```python
from build123d import *

# Parameters (mm, degrees)
SKETCH1_R           = 7.5
SKETCH1_R_2         = 4
BOSS_EXTRUDE1_DEPTH = 30
SKETCH4_R           = 2
CUT_EXTRUDE1_DEPTH  = 19


with BuildPart() as part:
    # Sketch1 → Boss-Extrude1 (new body)
    with BuildSketch(Plane.XY):
        Polygon((6.7, 11.09607963), (17, 11.09607963), (17, 5.09607963), (16.2, 3.09607963), (16.2, -5.843260198), (15.139339828, -6.90392037), (7.024607597, -6.90392037), (3.5, -10.90392037), (0, -10.90392037), (-3.5, -10.90392037), (-7.024607597, -6.90392037), (-15.139339828, -6.90392037), (-16.2, -5.843260198), (-16.2, 3.09607963), (-17, 5.09607963), (-17, 11.09607963), (-6.7, 11.09607963), (-6, 10.39607963), (6, 10.39607963), align=None)
        Circle(SKETCH1_R, mode=Mode.SUBTRACT)
        Circle(SKETCH1_R)
        Circle(SKETCH1_R_2, mode=Mode.SUBTRACT)
    extrude(amount=BOSS_EXTRUDE1_DEPTH)

    # Sketch4 → Cut-Extrude1 (cut, through all)
    with BuildSketch(Plane.XZ.offset(6.90392037)):
        with Locations((-12, 24)):
            Circle(SKETCH4_R)
        with Locations((-12, 6)):
            Circle(SKETCH4_R)
        with Locations((12, 6)):
            Circle(SKETCH4_R)
        with Locations((12, 24)):
            Circle(SKETCH4_R)
    extrude(amount=-CUT_EXTRUDE1_DEPTH, mode=Mode.SUBTRACT)


solid = part.part
```
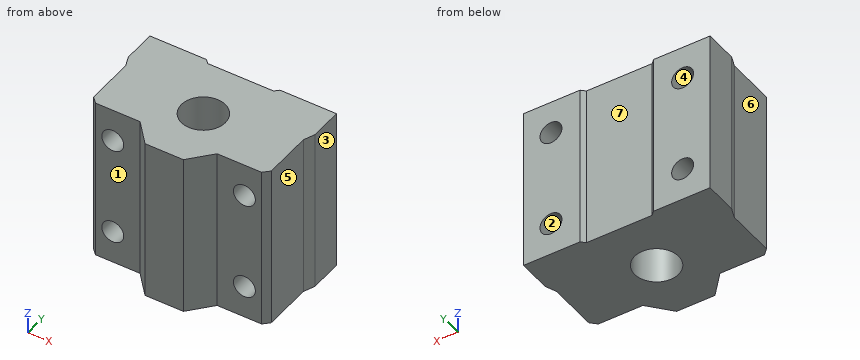
CAD build for the part. Positions are in the model's coordinates, mm. Face numbers are marked on the shaded views. A direction names the side the tool comes from. Round coordinates to 2 decimals unless told otherwise and drop trailing zeros. Loops run counter-clockwise (first coordinate to the right, second up) from the corner with the lowest first, then second, coordinate; pieces in that order, holes last. Notation, with made-up numbers: M 60,33.25 L 105,33.25 A17 ccw 105,59.25 Z; hole C 46,32 d2. An arc over 180 degrees is marked long. Return JSON: item names as keys, results as strings. Group by question number.
(1) Drop flat-ended pins along their axis: P1, Ø12, axis at y = -2.5, z = 6, coming from the +X side; P2, Ø2.5, axis at x = -10, z = 22, coming from the -Y side; P3, Ø1, axis at x = -1.5, z = 27, coming from the +Y side. Give the stop position or say it passes through.
(2) Saw through at D-D, the plane y = 7.75. List the corners of the cut face in (x, z), and give its area (3 significant figures).
(3) Mould opens along X. For the marked faces 1, 2, 3 and 4 say: +X half, -X half, draft (parallel to the pull), parting line (faces both ways), or undercut.
(4) Saw through at B-B, the plane y = 0. List the corners of the cut face in (x, z), and give its area (3 significant figures).
(5) Saw through at A-A, the plane z = 6. List the corners of the cut face in (x, y).
(6) Saw through at C-C, the plane x = 0. List the corners of the cut face in (y, z).
(7) Tool access for the marked faces 5, 6 and 7: list every direction of +Z, -Z, +X, -X, +Y, -Y with a clear straight run to the whole face (end or side of a thin tool).
(8) Wall check: probe 1 along Z at (x, y) = (-12, 7); probe 2 along Y at (x, z) = (0, 9.5); probe 3 along X at (y, z) = (-3.5, 25.5). Give the ranges that are in metal, low to high. Write a range as [from, to].
Answer list:
{
 "1": {"P1": "x = 16.36", "P2": "y = -6.9", "P3": "y = 10.4"},
 "2": {"outline": "M -17,0 L 17,0 L 17,30 L -17,30 Z; hole C -12,6 d4; hole C -12,24 d4; hole C 12,6 d4; hole C 12,24 d4", "area": "970 mm2"},
 "3": {"face 1": "draft", "face 2": "undercut", "face 3": "+X half", "face 4": "undercut"},
 "4": {"outline": "M -16.2,0 L -4,0 L -4,30 L -16.2,30 Z; M 4,0 L 16.2,0 L 16.2,30 L 4,30 Z; hole C -12,6 d4; hole C -12,24 d4; hole C 12,6 d4; hole C 12,24 d4", "area": "682 mm2"},
 "5": {"outline": "M -17,5.1 L -16.2,3.1 L -16.2,-5.84 L -15.14,-6.9 L -14,-6.9 L -14,11.1 L -17,11.1 Z; M -10,-6.9 L -7.02,-6.9 L -3.5,-10.9 L 3.5,-10.9 L 7.02,-6.9 L 10,-6.9 L 10,11.1 L 6.7,11.1 L 6,10.4 L -6,10.4 L -6.7,11.1 L -10,11.1 Z; M 14,-6.9 L 15.14,-6.9 L 16.2,-5.84 L 16.2,3.1 L 17,5.1 L 17,11.1 L 14,11.1 Z; hole C 0,0 d8"},
 "6": {"outline": "M -10.9,0 L -4,0 L -4,30 L -10.9,30 Z; M 4,0 L 10.4,0 L 10.4,30 L 4,30 Z"},
 "7": {"face 5": "+Z, -Z, +X, -Y", "face 6": "+Z, -Z, -X, -Y", "face 7": "+Z, -Z, +Y"},
 "8": {"probe 1": "[0, 4], [8, 22], [26, 30]", "probe 2": "[-10.9, -4], [4, 10.4]", "probe 3": "[-16.2, -13.32], [-10.68, -1.94], [1.94, 10.68], [13.32, 16.2]"}
}
